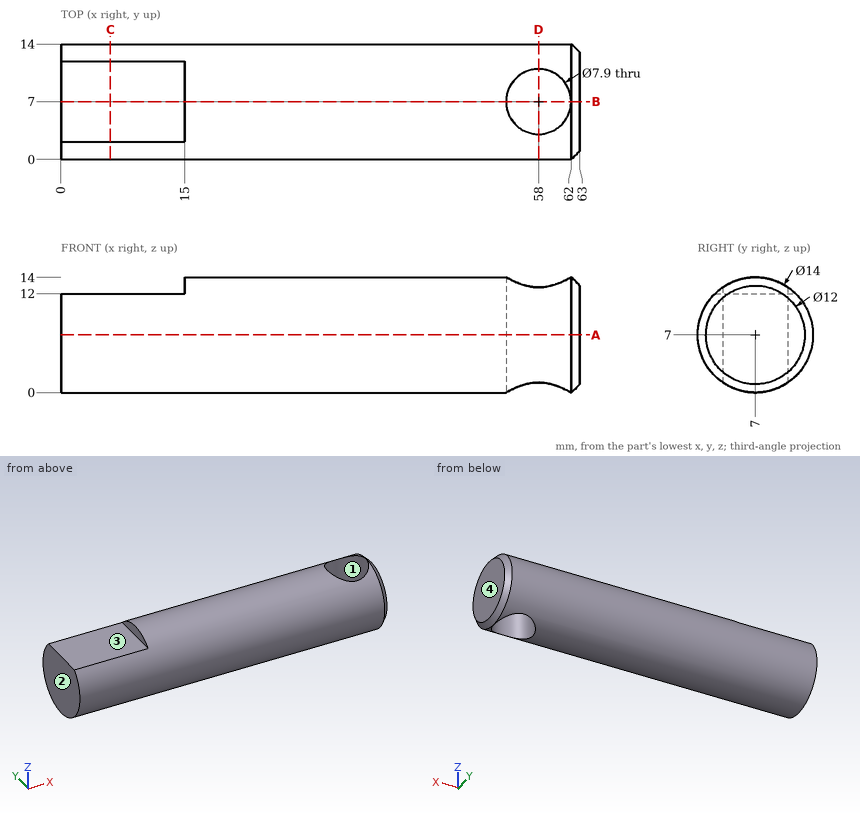
Here's the drawing with two shaded views (mm, measured from the low corner). I have some questions. Coordinates: 2 decimals unless noted, no trailing zeros. Loops run counter-clockwise (first coordinate to the right, second up) from the corner with the lowest first, then second, coordinate; pieces in that order, holes last. Notation, with made-up numbers: M 76,30.25 L 88,30.25 A22 cw 88,60.25 Z; hole C 75,43.25 d11. An arc over 180 degrees is marked long. Return JSON: item names as keys, results as strings. Group by question number.
Item 1: Thinking about a two-plate mould opening in X: for the marked faces 1, 2, 3 and 4, which applies, released by +X, released by -X, zero draft, split by the parting line, or undercut?
Item 2: I'm going to push flat-ended pins straight in: pin 1 Ø3 at (x, y) = (6, 8.5) entering from +Z; pin 2 Ø1.6 at (y, z) = (9.5, 13) entering from -X; pin 3 Ø5 at (x, y) = (55, 7) entering from -Z; pin 4 Ø4 at (x, y) = (27, 1.5) entering from +Z. Where does each tip first touch, or does it pass through?
Item 3: If I drill on L1, parallel to Y at x = 58, z = 3; L2, parallel to Y at x = 58, z = 6.25; L3, parallel to X at y = 9, z = 8.5, over which ranges is the centre line in solid material (lowest first)? Write a range as from..to.
Item 4: Imagine slicing it at B-B (y = 7). Please give me the cut outline in (x, z).
Item 5: Imagine slicing it at A-A (z = 7). Please give me the cut outline in (x, y).
Item 6: Imagine slicing it at D-D (x = 58). Please give me the cut outline in (y, z), and give its area (3 significant figures).
Item 7: Imagine slicing it at C-C (x = 6). Please give me the cut outline in (y, z).
Verdict:
{
 "1": {"face 1": "undercut", "face 2": "released by -X", "face 3": "zero draft", "face 4": "released by +X"},
 "2": {"pin 1": "stops at z = 12", "pin 2": "stops at x = 15", "pin 3": "stops at z = 0", "pin 4": "stops at z = 13.06"},
 "3": {"L1": "y = 1.26..3.05, 10.95..12.74", "L2": "y = 0.04..3.05, 10.95..13.96", "L3": "x = 0..54.59, 61.41..63"},
 "4": {"outline": "M 0,0 L 54.05,0 L 54.05,14 L 15,14 L 15,12 L 0,12 Z; M 61.95,0 L 62,0 L 63,1 L 63,13 L 62,14 L 61.95,14 Z"},
 "5": {"outline": "M 0,0 L 62,0 L 63,1 L 63,13 L 62,14 L 0,14 Z; hole C 58,7 d7.9"},
 "6": {"outline": "M 3.05,1.22 L 3.05,12.78 A7 ccw Z; M 10.95,1.22 A7 ccw 10.95,12.78 Z", "area": "49.5 mm^2"},
 "7": {"outline": "M 2.1,12 A7 ccw long 11.9,12 Z"}
}
